Check sheet for the modelled part. Datum: model origin and axes. Units: mm. A direction names the side the tool comes from. Coordinates: 2 decimals unless noted, no trailing zeros. Loops run counter-clockwise (first coordinate to the right, second up) from the corner with the lowest first, then second, coordinate; pieces in that order, holes last. Notation, with made-up numbers: (57.25, 8.25) - (68.25, 8.25) arc R29 cw to (68.25, 35.25) - close; hole circle Ø4 at (25, 74.25). An arc over 180 degrees is marked (long way). Use a Markdown table: item, result. Add a question column.
1) Go/stop test with a flat-tipped pin: P1, Ø5, axis at x = -0.5, y = 136.5, coming from the +Z side. Record where the tip stops, or that it passes through.
2) Sectioned sample at A-A, the plane z = 0. Enter the section's corners in (x, y) (3 decimals), then the cut area to 3 significant figures.
3) Thickness scan on line 1 (Z direction, x = -8, y = 131); line 2 (Z direction, x = 0, y = 104) (3 decimals). Record the ranges inside material, lowest first.
4) Draft check along Z on faces 4 (the flat face through (-3.655, 118, 0)), 5 (the flat face through (-10, 118, 6)), 6 (the flat face through (6, 118, 10)), 7 (the flat face through (0, 118, -3.655)). Enter one of: pulls with the +Z half, pulls with the -Z half, needs draft (parallel to the pull), parting line crosses it, or undercut.
5) Tool access check on faces 1 (the flat face through (0.1, 0, 2.4)), 2 (the flat face through (3.655, 118, 0)), 3 (the flat face through (0, 118, 3.655)). Record the directions out of +Z, -Z, +X, -X, +Y, -Y that give a thin tool (end or side, any length) a straight path to the whole face; none if there is none.
6) Sectioned sample at B-B, the plane x = 0. Enter the section's corners in (y, z) (3 decimals).
Autodesk Inventor part; units mm, degrees
ref_plane "YZ Plane" through (0, 0, 0) normal (1, 0, 0) x (0, 1, 0)
ref_plane "XZ Plane" through (0, 0, 0) normal (0, 1, 0) x (-1, 0, 0)
ref_plane "XY Plane" through (0, 0, 0) normal (0, 0, 1) x (1, 0, 0)
sketch "Sketch1" plane through (0, 0, 0) normal (0, 1, 0) x (-1, 0, 0)
  line L0 (0, -14) -> (0, 14)
  line L1 (-14, 0) -> (14, 0)
  line L2 (14, 0) -> (-14, 0)
  line L3 (0, -14) -> (0, 14)
  line L4 (2.5943, 3.655) -> (-2.5943, 3.655)
  line L5 (-3.655, 2.5943) -> (-3.655, -2.5943)
  line L6 (-2.5943, -3.655) -> (2.5943, -3.655)
  line L7 (3.655, -2.5943) -> (3.655, 2.5943)
  line L8 (-3.655, 3.655) -> (3.655, -3.655) construction
  line L9 (10, 10) -> (10, 2.63)
  line L10 (10, 2.63) -> (8.5, 2.63)
  line L11 (10, 10) -> (2.63, 10)
  line L12 (2.63, 10) -> (2.63, 8.5)
  line L13 (-10, 10) -> (-2.63, 10)
  line L14 (-2.63, 10) -> (-2.63, 8.5)
  line L15 (-10, 8.5) -> (-10, 10)
  line L16 (-10, 10) -> (-8.5, 10)
  line L17 (-8.5, 2.63) -> (-10, 2.63)
  line L18 (-10, 2.63) -> (-10, 10)
  line L19 (-10, -10) -> (-8.5, -10)
  line L20 (-8.5, -2.63) -> (-10, -2.63)
  line L21 (-10, -2.63) -> (-10, -10)
  line L22 (-10, -10) -> (-2.63, -10)
  line L23 (-2.63, -10) -> (-2.63, -8.5)
  line L24 (-10, -8.5) -> (-10, -10)
  line L25 (10, -10) -> (8.5, -10)
  line L26 (8.5, -2.63) -> (10, -2.63)
  line L27 (10, -2.63) -> (10, -10)
  line L28 (10, -10) -> (2.63, -10)
  line L29 (2.63, -10) -> (2.63, -8.5)
  line L30 (10, -8.5) -> (10, -10)
  circle A0 centre (0, 0) radius 2.095
  line L31 (5.995, -10) -> (2.63, -10)
  line L32 (-2.63, -10) -> (-5.995, -10)
  line L33 (10, -10) -> (2.63, -10)
  line L34 (-2.63, -10) -> (-10, -10)
  line L35 (10, -5.995) -> (10, -2.63)
  line L36 (10, 2.63) -> (10, 5.995)
  line L37 (10, 10) -> (10, 2.63)
  line L38 (10, -2.63) -> (10, -10)
  line L39 (-5.995, 10) -> (-2.63, 10)
  line L40 (2.63, 10) -> (5.995, 10)
  line L41 (-10, 10) -> (-2.63, 10)
  line L42 (2.63, 10) -> (10, 10)
  line L43 (-10, 5.995) -> (-10, 2.63)
  line L44 (-10, -2.63) -> (-10, -5.995)
  line L45 (-10, -10) -> (-10, -2.63)
  line L46 (-10, 2.63) -> (-10, 10)
  line L47 (-2.63, -8.5) -> (-5.995, -8.5)
  line L48 (-8.5, -5.995) -> (-8.5, -2.63)
  line L49 (-8.5, -5.995) -> (-7.0557, -5.995)
  line L50 (-5.995, -8.5) -> (-5.995, -7.0557)
  line L51 (-5.995, 7.0557) -> (-5.995, 8.5)
  line L52 (2.63, 8.5) -> (5.995, 8.5)
  line L53 (8.5, 2.63) -> (8.5, 5.995)
  line L54 (8.5, 5.995) -> (7.0557, 5.995)
  line L55 (5.995, 8.5) -> (5.995, 7.0557)
  line L56 (2.63, -8.5) -> (5.995, -8.5)
  line L57 (9.5607, -8.5) -> (10, -8.5)
  line L58 (8.5, -10) -> (8.5, -9.5607)
  line L59 (8.5, -5.995) -> (8.5, -2.63)
  line L60 (7.0557, -5.995) -> (8.5, -5.995)
  line L61 (5.995, -7.0557) -> (5.995, -8.5)
  line L62 (3.655, 3.655) -> (-0.5303, -0.5303) construction
  line L63 (-1.4814, -1.4814) -> (-3.655, -3.655) construction
  line L64 (-8.5, 10) -> (-8.5, 9.5607)
  line L65 (-8.5, 5.995) -> (-8.5, 2.63)
  line L66 (-2.63, 8.5) -> (-5.995, 8.5)
  line L67 (-9.5607, 8.5) -> (-10, 8.5)
  line L68 (-7.0557, 5.995) -> (-8.5, 5.995)
  line L69 (-3.655, 2.5943) -> (-7.0557, 5.995)
  line L70 (-2.5943, 3.655) -> (-5.995, 7.0557)
  line L71 (5.995, 7.0557) -> (2.5943, 3.655)
  line L72 (7.0557, 5.995) -> (3.655, 2.5943)
  line L73 (7.0557, -5.995) -> (3.655, -2.5943)
  line L74 (5.995, -7.0557) -> (2.5943, -3.655)
  line L75 (-2.5943, -3.655) -> (-5.995, -7.0557)
  line L76 (-3.655, -2.5943) -> (-7.0557, -5.995)
  dimension "d26" = 4.19
  dimension "d0" = 20
  dimension "d1" = 20
  dimension "d2" = 7.31
  dimension "d3" = 7.31
  dimension "d4" = 20
  dimension "d5" = 11.99
  dimension "d6" = 11.99
  dimension "d11" = 7.37
  dimension "d12" = 1.5
  dimension "d13" = 7.37
  dimension "d14" = 1.5
  dimension "d15" = 7.37
  dimension "d16" = 1.5
  dimension "d17" = 7.37
  dimension "d18" = 1.5
  dimension "d19" = 7.37
  dimension "d20" = 7.37
  dimension "d21" = 1.5
  dimension "d22" = 1.5
  dimension "d23" = 7.37
  dimension "d24" = 7.37
  dimension "d25" = 1.5
extrude "Extrusion1" add sketch "Sketch1" along normal blind 240 contours L6 L75 L50 L47 L23 L22 L19 L21 L20 L48 L49 L76 L5 L1 A0 L0 | L0 A0 L1 L7 L73 L60 L59 L26 L27 L25 L28 L29 L56 L61 L74 L6 | L1 L5 L69 L68 L65 L17 L18 L15 L13 L14 L66 L51 L70 L4 L0 A0 | A0 L0 L4 L71 L55 L52 L12 L11 L9 L10 L53 L54 L72 L7 L1
fillet "Fillet1" radius 0.5 20 edges at (10, 120, 10) (2.63, 120, 10) (-2.63, 120, 10) (-2.63, 120, 8.5) (10, 120, 2.63) (8.5, 120, 2.63) (10, 120, -2.63) (8.5, 120, -2.63) (10, 120, -10) (2.63, 120, -8.5) (-2.63, 120, -10) (-2.63, 120, -8.5) (2.63, 120, -10) (-10, 120, -10) (-8.5, 120, -2.63) (-10, 120, -2.63) (-8.5, 120, 2.63) (-10, 120, 2.63) (-10, 120, 10) (2.63, 120, 8.5)
fillet "Fillet2" radius 0.75 24 edges at (-7.0557, 120, 5.995) (-3.655, 120, 2.5943) (-8.5, 120, -5.995) (-7.0557, 120, -5.995) (-5.995, 120, -8.5) (3.655, 120, -2.5943) (7.0557, 120, -5.995) (-2.5943, 120, 3.655) (-5.995, 120, 7.0557) (3.655, 120, 2.5943) (7.0557, 120, 5.995) (8.5, 120, 5.995) (8.5, 120, -5.995) (2.5943, 120, 3.655) (5.995, 120, 7.0557) (5.995, 120, 8.5) (-5.995, 120, 8.5) (-8.5, 120, 5.995) (2.5943, 120, -3.655) (5.995, 120, -7.0557) (5.995, 120, -8.5) (-5.995, 120, -7.0557) (-2.5943, 120, -3.655) (-3.655, 120, -2.5943)
properties part number "Profile_Len_200mm"
Solved:
| question | item | result |
|---|---|---|
| 1 | P1 | stops at z = 9.98 |
| 2 | outline | (-3.655, 0) - (-2.095, 0) - (-2.095, 240) - (-3.655, 240) - close; (2.095, 0) - (3.655, 0) - (3.655, 240) - (2.095, 240) - close |
| 2 | area | 749 mm2 |
| 3 | line 1 | z = -10 to -5.95, 5.95 to 10 |
| 3 | line 2 | z = -3.655 to -2.095, 2.095 to 3.655 |
| 4 | face 4 | undercut |
| 4 | face 5 | needs draft |
| 4 | face 6 | pulls with the +Z half |
| 4 | face 7 | pulls with the -Z half |
| 5 | face 1 | +Z, -Z, +X, -X, -Y |
| 5 | face 2 | +X, +Y, -Y |
| 5 | face 3 | +Z, +Y, -Y |
| 6 | outline | (0, -3.655) - (240, -3.655) - (240, -2.095) - (0, -2.095) - close; (0, 2.095) - (240, 2.095) - (240, 3.655) - (0, 3.655) - close |
